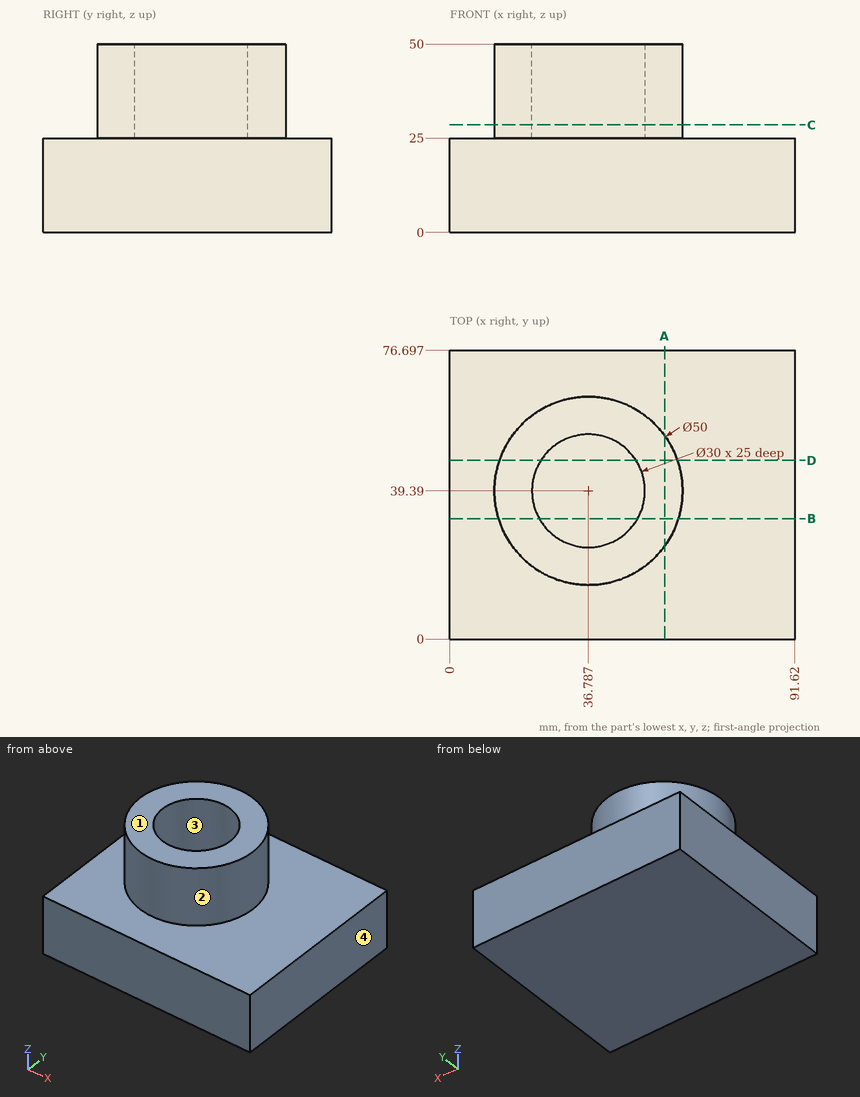
Drawing for the job (mm, zero at the part's lowest x, y, z). Coordinates: 2 decimals unless noted, no trailing zeros. Order: outer loops, then holes, each group sorted by start corner. A loop starts at its lowest first (then second) coordinate and runs counter-clockwise, first axis right, second up. Notation, with made-up numbers: (78.5, 57.5) -> (82.5, 57.5) arc R19 ccw to (82.5, 87.5) -> close; hole circle Ø5 at (-7.5, 28). An arc over 180 degrees is marked (long way). Return JSON: item names as keys, results as strings.
Item 1: Slice it at C-C (z = 28.5). Write the cut outline in (x, y).
Model answer:
{"outline": "circle Ø50 at (36.79, 39.39); hole circle Ø30 at (36.79, 39.39)"}
Item 2: Slice it at B-B (y = 32). Write the cut outline in (x, z).
Model answer:
{"outline": "(0, 0) -> (91.62, 0) -> (91.62, 25) -> (60.67, 25) -> (60.67, 50) -> (49.84, 50) -> (49.84, 25) -> (23.73, 25) -> (23.73, 50) -> (12.9, 50) -> (12.9, 25) -> (0, 25) -> close"}
Item 3: Pin check, flat tips, straight feed: P1, Ø1, axis at x = 10, z = 38, coming from the -Y side; P2, Ø10, axis at y = 43, z = 9, coming from the -X side; P3, Ø15, axis at x = 38, y = 45.5, coming from the +Z side; P4, Ø10, axis at y = 66.5, z = 44, coming from the -X side. Stop position of each tip, or through.
Model answer:
{"P1": "passes through", "P2": "stops at x = 0", "P3": "stops at z = 25", "P4": "stops at x = 25.12"}
Item 4: Mould opens along X. For the marked faces 1, 2, 3 and 4 say: pulls with the +X half, pulls with the -X half, needs draft (parallel to the pull), parting line crosses it, or undercut.
Model answer:
{"face 1": "needs draft", "face 2": "parting line crosses it", "face 3": "undercut", "face 4": "pulls with the +X half"}
Item 5: Slice it at D-D (y = 47.5). Write the cut outline in (x, z) (1 decimal), then the cut area to 3 significant figures.
Model answer:
{"outline": "(0, 0) -> (91.6, 0) -> (91.6, 25) -> (60.4, 25) -> (60.4, 50) -> (49.4, 50) -> (49.4, 25) -> (24.2, 25) -> (24.2, 50) -> (13.1, 50) -> (13.1, 25) -> (0, 25) -> close", "area": "2,840 mm²"}
Item 6: Wall check: line 1 along Z through (x, y) = (32.5, 33). Give the ranges that are in metal, low to high. Write a range as from..to.
Model answer:
{"line 1": "z = 0..25"}
Item 7: Slice it at A-A (x = 57). Write the cut outline in (y, z), then the cut area to 3 significant figures.
Model answer:
{"outline": "(0, 0) -> (76.7, 0) -> (76.7, 25) -> (54.1, 25) -> (54.1, 50) -> (24.68, 50) -> (24.68, 25) -> (0, 25) -> close", "area": "2,650 mm²"}
